Autodesk Inventor part; units mm, degrees
ref_plane "YZ Plane" through (0, 0, 0) normal (1, 0, 0) x (0, 1, 0)
ref_plane "XZ Plane" through (0, 0, 0) normal (0, 1, 0) x (-1, 0, 0)
ref_plane "XY Plane" through (0, 0, 0) normal (0, 0, 1) x (1, 0, 0)
sketch "Sketch1" plane through (0, 0, 0) normal (0, 1, 0) x (-1, 0, 0)
  line L0 (0, 0) -> (280, 0)
  line L1 (280, 0) -> (280, -280)
  line L2 (280, -280) -> (0, -280)
  line L3 (0, -280) -> (0, 0)
  line L4 (0, 0) -> (0, -20)
  line L5 (0, -20) -> (280, -20)
  line L6 (280, -20) -> (280, -260)
  line L7 (280, -260) -> (0, -260)
  line L8 (0, -260) -> (0, -20)
  dimension "d0" = 280
  dimension "d1" = 280
  dimension "d2" = 20
  dimension "d3" = 240
extrude "Extrusion1" add sketch "Sketch1" along normal blind 244 contours L5 L1 L7 L3
sketch "Sketch2" plane through (0, 0, 0) normal (0, -1, 0) x (1, 0, 0)
  line L0 (0, 0) -> (-280, 0)
  line L1 (-280, 0) -> (-280, -280)
  line L2 (-280, -280) -> (0, -280)
  line L3 (0, -280) -> (0, 0)
  dimension "d6" = 280
  dimension "d7" = 280
extrude "Extrusion2" add sketch "Sketch2" against normal blind 40
sketch "Sketch3" plane through (-280, 244, -20) normal (0, 0, 1) x (1, 0, 0)
  line L0 (0, -244) -> (280, -244)
  line L1 (0, -244) -> (0, -80)
  line L2 (0, -204) -> (0, 0)
  line L3 (0, 0) -> (80, 0)
  line L4 (0, 0) -> (280, 0)
  line L5 (80, 0) -> (130, 0)
  line L6 (280, -244) -> (280, -150)
  line L7 (280, -244) -> (280, -204)
  line L8 (280, -150) -> (130, 0)
  line L9 (0, -80) -> (80, 0)
  line L10 (0, 0) -> (0, -80)
  line L11 (280, 0) -> (280, -150)
  line L12 (280, 0) -> (130, 0)
  dimension "d10" = 164
  dimension "d11" = 80
  dimension "d12" = 50
  dimension "d13" = 94
extrude "Extrusion3" cut sketch "Sketch3" against normal through all contours L2 L3 L9 | L8 L4 L11
sketch "Sketch4" plane through (-150, 244, -260) normal (0.7071, 0.7071, 0) x (-0.7071, 0.7071, 0)
  line L0 (-212.132, 0) -> (-212.132, 240)
  line L1 (-212.132, 240) -> (0, 240)
  point P0 (-278.6001, 260)
  point P1 (-112.132, 120)
  dimension "d16" = 100
  dimension "d17" = 120
hole "Hole1" at (-70.7107, 164.7107, -140) direction (-0.7071, -0.7071, 0) diameter 150 end through all
sketch "Sketch5" plane through (-280, 40, -20) normal (0, 0, 1) x (1, 0, 0)
  line L0 (280, 0) -> (0, 0)
  line L1 (0, 0) -> (280, 0)
  line L2 (130, 204) -> (280, 54)
  line L3 (280, 0) -> (280, 54)
  line L4 (280, 54) -> (130, 204)
  line L5 (130, 204) -> (80, 204)
  line L6 (130, 204) -> (80, 204)
  line L7 (0, 0) -> (0, 124)
  line L8 (80, 204) -> (0, 124)
  line L9 (0, 124) -> (0, 0)
  point P0 (280, -40)
extrude "Extrusion4" cut sketch "Sketch5" against normal blind 20
sketch "Sketch6" plane through (0, 40, -260) normal (0, 0, -1) x (-1, 0, 0)
  line L0 (0, 0) -> (280, 0)
  line L1 (150, 204) -> (0, 54)
  line L2 (0, 0) -> (0, 54)
  line L3 (0, 54) -> (150, 204)
  line L4 (280, 124) -> (200, 204)
  line L5 (150, 204) -> (200, 204)
  line L6 (200, 204) -> (280, 124)
  line L7 (280, 124) -> (280, 0)
  line L8 (280, 0) -> (0, 0)
  point P0 (0, -40)
extrude "Extrusion5" cut sketch "Sketch6" against normal blind 20
properties part number "MMAE 232 - Assignment 1a-Nicholas Skiba" material "Aluminum 6061"
Input: part model. Units: mm. Frame: model coordinates. A direction names the side the tool comes from. Give positions to 0.01 mm unless a question says otherwise; leave off trailing zeros. Order: outer loops, then holes, each group sorted by start corner. A loop starts at its lowest first (then second) coordinate and runs counter-clockwise, first axis right, second up. Notation, with made-up numbers: (79, 36.5) - (125, 36.5) arc R20 cw to (125, 46.5) - close; hole circle Ø8 at (-28, 45.5). An arc over 180 degrees is marked (long way). Write each question's results on one line, items separated by ' | '.
Item 1: Section A-A (z = -149.5). Return loops of the section in (x, y), and give its area (3 significant figures).
A:
outline: (-280, 60.63) - (-123.32, 217.32) - (-150, 244) - (-200, 244) - (-280, 164) - close; (-130.21, 0) - (0, 0) - (0, 94) - (-18.1, 112.1) - close | area: 21,000 mm^2
Item 2: Access query for faces 5 (the flat face through (-138, 40, -20)), 6 (the flat face through (0, 46, -142)), 7 (the flat face through (-169, 121, -240)). Directions: +Z, -Z, +X, -X, +Y, -Y. A direction counts if a zero-diameter tool reaches every point of the face in a straight line with its end or side. Return the directions, or none.
A:
face 5: +Z, +X, -X, +Y | face 6: +Z, -Z, +X, +Y, -Y | face 7: -Z, +X, -X, +Y
Item 3: Section B-B (z = -225). Return loops of the section in (x, y).
A:
outline: (-280, 0) - (0, 0) - (0, 94) - (-150, 244) - (-200, 244) - (-280, 164) - close
Item 4: Section C-C (z = -86). Return loops of the section in (x, y), and give its area (3 significant figures).
A:
outline: (-280, 29.03) - (-107.51, 201.51) - (-150, 244) - (-200, 244) - (-280, 164) - close; (-161.81, 0) - (0, 0) - (0, 94) - (-33.91, 127.91) - close | area: 30,000 mm^2
Item 5: Contact query for flat-ended pins moving along their axis: pin 1 Ø1 at (y, z) = (185.5, -98.5) entering from +X; pin 2 Ø8 at (x, z) = (-211.5, -250) entering from +Y; pin 3 Ø4 at (y, z) = (171, -84) entering from -X. Output: stop coordinate, or through.
A:
pin 1: stops at x = -137.58 | pin 2: stops at y = 40 | pin 3: stops at x = -275
Item 6: Material intervals for line 1 along Z through (x, y) = (-157, 143); line 2 along Z through (x, y) = (-87.5, 56); line 3 along Y through (x, z) = (-139, -104), sorted ascending.
A:
line 1: z = -240 to -199.5, -80.5 to -40 | line 2: z = -240 to -177.42, -102.58 to -40 | line 3: y = 0 to 3.37, 189.47 to 233
Item 7: Section D-D (z = -18.5). Return loops of the section in (x, y).
A:
outline: (-280, 0) - (0, 0) - (0, 40) - (-280, 40) - close
Item 8: Draft query along Y for faces 1 (the flat face through (-175, 244, -139)), 2 (the flat face through (-138, 20, 0)), 3 (the cylindrical face through (-189.46, 135.397, -99.68)), 4 (the flat face through (-107, 0, -138)). Return one class per face: released by +Y, released by -Y, zero draft, split by the parting line, or undercut.
A:
face 1: released by +Y | face 2: zero draft | face 3: undercut | face 4: released by -Y
